Autodesk Inventor part; units mm, degrees
ref_plane "WorkPlane1" through (0, 0, 0) normal (0, 0, 1) x (1, 0, 0)
ref_plane "Work Plane2" through (0, 0, -1) normal (0, 0, 1) x (1, 0, 0)
ref_plane "WorkPlane2" through (0, 0, 1) normal (0, 0, 1) x (1, 0, 0)
ref_plane "WorkPlane1" through (0, 0, 0) normal (0, 0, 1) x (1, 0, 0)
ref_plane "Work Plane2" through (0, 0, -1) normal (0, 0, 1) x (1, 0, 0)
ref_plane "WorkPlane2" through (0, 0, 1) normal (0, 0, 1) x (1, 0, 0)
sketch "Sketch1" plane through (0, 0, 0) normal (0, 0, 1) x (1, 0, 0)
  point P0 (0, 0)
sketch "Sketch2" plane through (0, 0, 0) normal (0, 0, 1) x (1, 0, 0)
  line L0 (4.42, -6.7764) -> (3.4917, -5.2763)
  arc A0 (5.3722, -3.0552) -> (3.4917, -5.2763) centre (4.7928, -4.4712) ccw
  line L1 (5.3722, -3.0552) -> (6.3125, -3.4399)
  arc A1 (6.3125, -3.4399) -> (-6.3125, -3.4399) centre (0, 0) ccw
  line L2 (-5.3722, -3.0552) -> (-6.3125, -3.4399)
  arc A2 (-3.4917, -5.2763) -> (-5.3722, -3.0552) centre (-4.7928, -4.4712) ccw
  line L3 (-4.42, -6.7764) -> (-3.4917, -5.2763)
  arc A3 (4.42, -6.7764) -> (-4.42, -6.7764) centre (0, 0.3667) ccw
  line L4 (0, 0.3667) -> (-4.42, -6.7764) construction
  line L5 (0, 0.3667) -> (4.42, -6.7764) construction
  dimension "d2" = 8.4
  dimension "d4" = 0
  dimension "d6" = 7.1889
  dimension "d8" = 0.3667
  dimension "d10" = 4.42
  dimension "d12" = 4.42
  dimension "d14" = 1.53
  dimension "d16" = 1.53
  dimension "d18" = 6.81
  dimension "d20" = 6.81
  dimension "d22" = 36
  dimension "d24" = 36
extrude "Extrusion1" add sketch "Sketch2" along normal blind 1
sketch "Sketch3" plane through (0, 0, 1) normal (0, 0, 1) x (1, 0, 0)
  arc A0 (-3.4917, -5.2763) -> (-5.3722, -3.0552) centre (-4.7928, -4.4712) ccw
hole "Hole1" at (-4.7928, -4.4712, 1) direction (0, 0, -1) diameter 1.7 end through all
sketch "Sketch4" plane through (0, 0, 1) normal (0, 0, 1) x (1, 0, 0)
  arc A0 (5.3722, -3.0552) -> (3.4917, -5.2763) centre (4.7928, -4.4712) ccw
hole "Hole2" at (4.7928, -4.4712, 1) direction (0, 0, -1) diameter 1.7 end through all
equation "\"d29\" = Diam5"
equation "\"d36\" = Diam5"
equation "\"d2\" = 0.5 * Diam2"
equation "\"d6\" = 0.5 * msp_dd1"
equation "\"d8\" = -0.5 * msp_dd1 + 0.5 * Diam2 - 0.222222 * ParA"
equation "\"d10\" = 2.6 * Diam5"
equation "\"d12\" = 2.6 * Diam5"
equation "\"d14\" = 0.9 * Diam5"
equation "\"d16\" = 0.9 * Diam5"
equation "\"d18\" = 1.3 * Diam5 + 0.5 * Diam2 - ParA"
equation "\"d20\" = 1.3 * Diam5 + 0.5 * Diam2 - ParA"
equation "\"d25\" = ParS"
equation "\"Diam5\" = 1.7"
equation "\"ParA\" = 3.8"
equation "\"ParS\" = 1"
equation "\"Diam2\" = 16.8"
equation "\"msp_dd1\" = -b + Diam2 - 0.111111 * ParA"
equation "\"msp_pom\" = 0.5 * Diam2 - b"
equation "\"TEMPLATE\" = 1.2345"
properties part number "DIN 472 - 16x1" material "Steel, Mild"
The model under review builds one solid part; all positions refer to its coordinate system, in mm. A direction names the side the tool comes from. Give positions to 0.01 mm unless a question says otherwise; leave off trailing zeros. Write each loop counter-clockwise with the first axis right and the second up, starting at its lowest first coordinate (ties: lowest second). Pieces come first, ordered by that corner, then holes.
1. Add section D-D, the plane x = -7. Write out the cut boundary in (y, z), plus the area to 3 significant figures.
2. Add section C-C, the plane z = 0.15. Write out the cut boundary in (x, y).
3. For P1, Ø8, axis at x = 3.5, y = -3, coming from the +Z side, flat-tipped, find the tip position at first contact; note if it passes through.
4. Add section B-B, the plane y = 3. Write out the cut boundary in (x, z), plus the area to 3 significant figures.
5. Draft analysis for pull direction Y (two halves, no side actions). For faces 4 (the cylindrical face through (-4.467, -5.256, 0.493)), 5 (the flat face through (-3.962, -6.037, 0.493)), 6 (the flat face through (-5.836, -3.245, 0.493)), 7 (the flat face through (0, 7.4, 0)), state which applies: +Y half, -Y half, draft (parallel to the pull), parting line (faces both ways), or undercut.
6. Add section A-A, the plane y = -5. Write out the cut boundary in (x, z), plus the area to 3 significant figures.
7. Wall thickness on L1, parallel to Y at x = 4.25, z = 0.85; L2, parallel to X at y = -3.25, z = 0.75; L3, parallel to X at y = -4, z = 0.9: over which ranges is each line inside the solid? List them lowest first.
8. Tool access review of faces 1 (the flat face through (0, 7.4, 1)), 2 (the flat face through (5.836, -3.245, 0.493)), 3 (the flat face through (3.962, -6.037, 0.493)): name each direction out of +Z, -Z, +X, -X, +Y, -Y from which nothing blocks a thin tool from reaching the whole face with its end or side.
Worked answers:
1. outline: (-4.28, 0) - (-1.64, 0) - (-1.64, 1) - (-4.28, 1) - close; (1.64, 0) - (5.01, 0) - (5.01, 1) - (1.64, 1) - close
1. area: 6.01 mm2
2. outline: (-6.31, -3.44) arc R7.19 cw (long way) to (6.31, -3.44) - (5.37, -3.06) arc R1.53 ccw to (3.49, -5.28) - (4.42, -6.78) arc R8.4 ccw (long way) to (-4.42, -6.78) - (-3.49, -5.28) arc R1.53 ccw to (-5.37, -3.06) - close; hole circle Ø1.7 at (-4.79, -4.47); hole circle Ø1.7 at (4.79, -4.47)
3. P1: stops at z = 1
4. outline: (-7.98, 0) - (-6.53, 0) - (-6.53, 1) - (-7.98, 1) - close; (6.53, 0) - (7.98, 0) - (7.98, 1) - (6.53, 1) - close
4. area: 2.89 mm2
5. face 4: undercut
5. face 5: -Y half
5. face 6: undercut
5. face 7: draft
6. outline: (-6.46, 0) - (-5.46, 0) - (-5.46, 1) - (-6.46, 1) - close; (-4.13, 0) - (-3.36, 0) - (-3.36, 1) - (-4.13, 1) - close; (3.36, 0) - (4.13, 0) - (4.13, 1) - (3.36, 1) - close; (5.46, 0) - (6.46, 0) - (6.46, 1) - (5.46, 1) - close
6. area: 3.55 mm2
7. L1: y = -6.5 to -5.13, -3.82 to -3.04, 5.8 to 7.61
7. L2: x = -7.58 to -6.41, -5.85 to -3.87, 3.87 to 5.85, 6.41 to 7.58
7. L3: x = -7.18 to -5.5, -4.09 to -3.34, 3.34 to 4.09, 5.5 to 7.18
8. face 1: +Z, +X, -X, +Y, -Y
8. face 2: +Z, -Z
8. face 3: +Z, -Z, -Y
